```python
from build123d import *

# Parameters (mm, degrees)
SKETCH1_R           = 60
BOSS_EXTRUDE1_DEPTH = 5
CUT_EXTRUDE1_DEPTH  = 5
BOSS_EXTRUDE2_DEPTH = 23
SKETCH4_R           = 2.25
CUT_EXTRUDE2_DEPTH  = 15
BOSS_EXTRUDE3_START = -5
BOSS_EXTRUDE3_DEPTH = 5
SKETCH10_R          = 14
BOSS_EXTRUDE6_DEPTH = 3


with BuildPart() as part:
    # Sketch1 → Boss-Extrude1 (new body)
    with BuildSketch(Plane(origin=(0, 0, 0), x_dir=(1, 0, 0), z_dir=(0, 1, 0))):
        with Locations(Location((0, 0, 0), (0, 0, 270))):
            Circle(SKETCH1_R)
    extrude(amount=BOSS_EXTRUDE1_DEPTH)

    # Sketch2 → Cut-Extrude1 (cut)
    with BuildSketch(Plane(origin=(0, 5, 0), x_dir=(1, 0, 0), z_dir=(0, 1, 0))):
        with BuildLine():
            ThreePointArc((-43.005482325, 30.112762908), (-52.5, 0), (-43.005482325, -30.112762908))
            ThreePointArc((-43.005482325, -30.112762908), (-29.078197519, -32.568518988), (-26.622441439, -18.641234181))
            ThreePointArc((-26.622441439, -18.641234181), (-32.5, 0), (-26.622441439, 18.641234181))
            ThreePointArc((-26.622441439, 18.641234181), (-29.078197519, 32.568518988), (-43.005482325, 30.112762908))
        make_face()
        with BuildLine():
            ThreePointArc((43.005482325, 30.112762908), (29.078197519, 32.568518988), (26.622441439, 18.641234181))
            ThreePointArc((26.622441439, 18.641234181), (32.5, 0), (26.622441439, -18.641234181))
            ThreePointArc((26.622441439, -18.641234181), (29.078197519, -32.568518988), (43.005482325, -30.112762908))
            ThreePointArc((43.005482325, -30.112762908), (52.5, 0), (43.005482325, 30.112762908))
        make_face()
    extrude(amount=-CUT_EXTRUDE1_DEPTH, mode=Mode.SUBTRACT)

    # Sketch3 → Boss-Extrude2 (add)
    with BuildSketch(Plane(origin=(0, 5, 0), x_dir=(1, 0, 0), z_dir=(0, 1, 0))):
        with BuildLine():
            Line((10, 56.623758265), (10, 59.160797831))
            ThreePointArc((10, 59.160797831), (0, 60), (-10, 59.160797831))
            Line((-10, 59.160797831), (-10, 56.623758265))
            Line((-10, 56.623758265), (10, 56.623758265))
        make_face()
    extrude(amount=BOSS_EXTRUDE2_DEPTH)

    # Sketch4 → Cut-Extrude2 (cut)
    with BuildSketch(Plane(origin=(0, 5, 0), x_dir=(1, 0, 0), z_dir=(0, 1, 0))):
        with Locations(Location((0, 0, 0), (0, 0, 270))):
            Circle(SKETCH4_R)
    extrude(amount=-CUT_EXTRUDE2_DEPTH, mode=Mode.SUBTRACT)

    # Sketch5 → Boss-Extrude3 (add)
    with BuildSketch(Plane(origin=(0, 5, 0), x_dir=(1, 0, 0), z_dir=(0, 1, 0)).offset(BOSS_EXTRUDE3_START)):
        with BuildLine():
            Line((-58.094750193, 15), (-158.094750193, 15))
            Line((-158.094750193, 15), (-158.094750193, -15))
            Line((-158.094750193, -15), (-58.094750193, -15))
            ThreePointArc((-58.094750193, -15), (-60, 0), (-58.094750193, 15))
        make_face()
    boss_extrude3 = extrude(amount=BOSS_EXTRUDE3_DEPTH)

    # Mirror1: Boss-Extrude3 across plane
    add(boss_extrude3.mirror(Plane(origin=(0, 0, 0), x_dir=(0, 0, 1), z_dir=(1, 0, 0))))

    # Sketch10 → Boss-Extrude6 (add)
    with BuildSketch(Plane(origin=(0, 28, 0), x_dir=(1, 0, 0), z_dir=(0, 1, 0))):
        with BuildLine():
            Line((-10, 59.160797831), (-10, 56.623758265))
            ThreePointArc((-10, 56.623758265), (0, 25.41910773), (10, 56.623758265))
            Line((10, 56.623758265), (10, 59.160797831))
            Line((10, 59.160797831), (0, 60))
            Line((0, 60), (-10, 59.160797831))
        make_face()
        with Locations(Location((0, 42.623758265, 0), (0, 0, 90))):
            Circle(SKETCH10_R, mode=Mode.SUBTRACT)
    extrude(amount=BOSS_EXTRUDE6_DEPTH)


solid = part.part
```
The model under review builds one solid part; all positions refer to its coordinate system, in mm. A direction names the side the tool comes from. Round coordinates to 2 decimals unless told otherwise and drop trailing zeros. Loops run counter-clockwise (first coordinate to the right, second up) from the corner with the lowest first, then second, coordinate; pieces in that order, holes last.
1) Tool access review of faces 5 (the face through (0, 7, -60)), 6 (the face through (-52.5, 2.5, -0.4)), 7 (the face through (0, 16, -56.624)): name each direction out of +Z, -Z, +X, -X, +Y, -Y from which nothing blocks a thin tool from reaching the whole face with its end or side.
Values follow:
face 5: -Z, +Y, -Y
face 6: +Y, -Y
face 7: +Z, +X, -X
2) Wall thickness on line 1 along X through (y, z) = (2.1, 0); line 2 along X through (y, z) = (4.5, -23); line 3 along Y through (x, z) = (2.5, 27): over which ranges is each line inside the solid? List them lowest first.
Values follow:
line 1: x = -158.09 to -52.5, -32.5 to -2.25, 2.25 to 32.5, 52.5 to 158.09
line 2: x = -55.42 to -47.19, -24.91 to 24.91, 47.19 to 55.42
line 3: y = 0 to 5
3) Clearance check with flat-ended pins moving along their axes: P1, Ø0.8, axis at y = 14, z = -57.5, coming from the -X side; P2, Ø6, axis at y = 6.5, z = 31.5, coming from the -X side; P3, Ø12, axis at x = -4, z = -2.5, coming from the +Y side; P4, Ø4, axis at x = 58, y = 8, coming from the -Z side. State where each tip first meets the part, or that it passes through.
Values follow:
P1: stops at x = -10
P2: stops at x = -52.58
P3: stops at y = 5
P4: passes through
4) The part is to be moulded in two halves that separate along X. For faces 1 (the face through (28.9, 2.54, 32.44)), 2 (the face through (-0.616, 29.479, -28.637)), 3 (the face through (-0.61, 29.48, -25.43)), 4 (the face through (0, 31, -57)), say which applies: pulls with the +X half, pulls with the -X half, needs draft (parallel to the pull), parting line crosses it, or undercut.
Values follow:
face 1: undercut
face 2: undercut
face 3: parting line crosses it
face 4: needs draft
5) Consider section B-B on y = 18.5. State the section outline as (x, z) points.
Values follow:
outline: (-10, -59.16) arc R60 ccw to (10, -59.16) - (10, -56.62) - (-10, -56.62) - close
6) Consider section A-A on z = -9. State the section outline as (x, y) points.
Values follow:
outline: (-158.09, 0) - (-51.72, 0) - (-51.72, 5) - (-158.09, 5) - close; (-31.23, 0) - (31.23, 0) - (31.23, 5) - (-31.23, 5) - close; (51.72, 0) - (158.09, 0) - (158.09, 5) - (51.72, 5) - close
